Build history of the part. All positions in model axes, mm. A direction names the side the tool comes from. Round coordinates to 2 decimals unless told otherwise and drop trailing zeros. Write each loop counter-clockwise with the first axis right and the second up, starting at its lowest first coordinate (ties: lowest second). Pieces come first, ordered by that corner, then holes. Notation, with made-up numbers: (89.5, 34.25) -> (137.5, 34.25) arc R20 ccw to (137.5, 62.25) -> close; hole circle Ø1 at (80.5, 32). An arc over 180 degrees is marked (long way). Answer as CSV lines item,"result".
from build123d import *

# Parameters (mm, degrees)
SALIENTE_EXTRUIR1_DEPTH = 9.08
SALIENTE_EXTRUIR4_DEPTH = 1.5
SALIENTE_EXTRUIR5_DEPTH = 4.08


with BuildPart() as part:
    # Croquis1 → Saliente-Extruir1 (new body)
    with BuildSketch(Plane.XY):
        Polygon((126.24514053, -55.999935), (126.24514053, -50.999935), (121.99984, -50.999935), (113.25453947, -59.74523553), (113.25453947, -64.74523553), (115.25453947, -62.74523553), (115.25453947, -60.24523553), (119.25453947, -56.24523553), (119.25453947, -58.74523553), (121.99984, -55.999935), align=None)
    extrude(amount=-SALIENTE_EXTRUIR1_DEPTH)

    # Croquis4 → Saliente-Extruir4 (add)
    with BuildSketch(Plane.XY):
        Polygon((115.25453947, -60.24523553), (115.25453947, -62.74523553), (119.25453947, -58.74523553), (119.25453947, -56.24523553), align=None)
    extrude(amount=-SALIENTE_EXTRUIR4_DEPTH)

    # Croquis5 → Saliente-Extruir5 (add)
    with BuildSketch(Plane(origin=(0, 0, -9.08), x_dir=(-1, 0, 0), z_dir=(0, 0, -1))):
        Polygon((-115.25453947, -60.24523553), (-115.25453947, -62.74523553), (-119.25453947, -58.74523553), (-119.25453947, -56.24523553), align=None)
    extrude(amount=-SALIENTE_EXTRUIR5_DEPTH)


solid = part.part
1. Mould opens along X. For faces 6 (the flat face through (113.255, -62, -4)), 7 (the flat face through (120, -56, 0)), 8 (the flat face through (117, -59, -1.5)) say: +X half, -X half, draft (parallel to the pull), parting line (faces both ways), or undercut.
Results found:
face 6,"-X half"
face 7,"draft"
face 8,"undercut"
2. Probe line 1 along Y through (x, z) = (124, -2.5); line 2 along X through (y, z) = (-62.75, -0.5); line 3 along X through (y, z) = (-53.75, -2.5). List the from-to ranges inside material, lowest first.
Results found:
line 1,"y = -56 to -51"
line 2,"x = 113.25 to 115.25"
line 3,"x = 119.25 to 126.25"
3. Drop flat-ended pins along their axis: pin 1 Ø1.5 at (x, z) = (116, -2) entering from +Y; pin 2 Ø1.2 at (x, y) = (117.5, -58.5) entering from +Z; pin 3 Ø1.3 at (x, z) = (125, -4) entering from -Y; pin 4 Ø4 at (y, z) = (-53.5, -7.5) entering from -X. Give the stop position or say it passes through.
Results found:
pin 1,"stops at y = -56.25"
pin 2,"stops at z = 0"
pin 3,"stops at y = -56"
pin 4,"stops at x = 117.5"
4. Cut at B-B, the plane y = -56.75. Write the cut outline in (x, z).
Results found:
outline,"(116.25, -9.08) -> (121.25, -9.08) -> (121.25, 0) -> (116.25, 0) -> close; hole (118.75, -5) -> (119.25, -5) -> (119.25, -1.5) -> (118.75, -1.5) -> close"
5. Cut at A-A, the plane z = -2.25. Write the cut outline in (x, y), then the cut area to 3 significant figures.
Results found:
outline,"(113.25, -64.75) -> (115.25, -62.75) -> (115.25, -60.25) -> (119.25, -56.25) -> (119.25, -58.75) -> (122, -56) -> (126.25, -56) -> (126.25, -51) -> (122, -51) -> (113.25, -59.75) -> close"
area,"55.0 mm2"
6. Which spindle directions (+Z, -Z, +X, -X, +Y, -Y) get a long thin tool onto all of the face, cutting with end or side? Do faces 1 (the flat face through (115.255, -62, -3)), 2 (the flat face through (124, -56, -4)), 3 (the flat face through (124, -51, -4)), 4 (the flat face through (120, -56, -9.08)), 5 (the flat face through (117.2, -58.3, -3.2)). Say none if no direction does.
Results found:
face 1,"+X, -Y"
face 2,"+Z, -Z, +X, -Y"
face 3,"+Z, -Z, +X, -X, +Y"
face 4,"-Z, +X, -X, +Y, -Y"
face 5,"-Y"
7. Cut at C-C, the plane x = 117.75. Write the cut outline in (y, z).
Results found:
outline,"(-60.25, -9.08) -> (-55.25, -9.08) -> (-55.25, 0) -> (-60.25, 0) -> (-60.25, -1.5) -> (-57.75, -1.5) -> (-57.75, -5) -> (-60.25, -5) -> close"
8. Cut at D-D, the plane y = -60.75. Write the cut outline in (x, z), then the cut area to 3 significant figures.
Results found:
outline,"(113.25, -9.08) -> (117.25, -9.08) -> (117.25, -5) -> (115.25, -5) -> (115.25, -1.5) -> (117.25, -1.5) -> (117.25, 0) -> (113.25, 0) -> close"
area,"29.3 mm2"
